Can you work these out from the model? Positions are in its coordinate system, mm. Give positions to 0.01 mm unless a question says otherwise; leave off trailing zeros. Order: outer loops, then holes, each group sorted by start corner. A loop starts at its lowest first (then second) coordinate and runs counter-clockwise, first axis right, second up. Notation, with made-up numbers: (51, 2.25) -> (66, 2.25) arc R14 cw to (66, 15.25) -> close; hole circle Ø11 at (33.5, -26). An arc over 180 degrees is marked (long way). Answer as a JSON object with one key per item and string values.
```python
from build123d import *

# Parameters (mm, degrees)
SKETCH_1_R          = 1.5
EXTRUDE_1_DEPTH     = 2
FILLET_2_R          = 5
FILLET_3_R          = 5
SKETCH_7_R          = 6
CUT_EXTRUDE_4_DEPTH = 10
FILLET_5_R          = 5
SKETCH_8_W          = 10
SKETCH_8_H          = 2
EXTRUDE_3_DEPTH     = 12
SKETCH_9_R          = 1.5
CUT_EXTRUDE_5_DEPTH = 12
FILLET_6_R          = 2
SKETCH_10_W         = 10
SKETCH_10_H         = 2
EXTRUDE_4_DEPTH     = 14
FILLET_7_R          = 5
FILLET_8_R          = 5


with BuildPart() as part:
    # 草图1 → 凸台-拉伸1 (new body)
    with BuildSketch(Plane(origin=(0, 0, 0), x_dir=(1, 0, 0), z_dir=(0, 1, 0))):
        with BuildLine():
            Line((17.196152423, -13), (52, -13))
            Line((52, -13), (52, -5.5))
            Line((52, -5.5), (-15, -5.5))
            Line((-15, -5.5), (-15, 5))
            Line((-15, 5), (-25, 5))
            Line((-25, 5), (-25, -13))
            Line((-25, -13), (6.803847577, -13))
            ThreePointArc((6.803847577, -13), (12, -16), (17.196152423, -13))
        make_face()
        with Locations(Location((-20, 0, 0), (0, 0, 270))):
            Circle(SKETCH_1_R, mode=Mode.SUBTRACT)
    extrude(amount=EXTRUDE_1_DEPTH)

    # 圆角2
    fillet_2_edges = [part.edges().sort_by_distance(p)[0] for p in [
        (-25, 1, -5),
    ]]
    fillet(fillet_2_edges, radius=FILLET_2_R)

    # 圆角3
    fillet_3_edges = [part.edges().sort_by_distance(p)[0] for p in [
        (-25, 1, 13),
    ]]
    fillet(fillet_3_edges, radius=FILLET_3_R)

    # 草图7 → 切除-拉伸4 (cut)
    with BuildSketch(Plane(origin=(0, 2, 0), x_dir=(1, 0, 0), z_dir=(0, 1, 0))):
        with Locations((12, -2.5)):
            Circle(SKETCH_7_R)
    extrude(amount=-CUT_EXTRUDE_4_DEPTH, mode=Mode.SUBTRACT)

    # 圆角5
    fillet_5_edges = [part.edges().sort_by_distance(p)[0] for p in [
        (17.196152423, 1, 13),
        (6.803847577, 1, 13),
        (6.803847577, 1, 5.5),
        (17.196152423, 1, 5.5),
    ]]
    fillet(fillet_5_edges, radius=FILLET_5_R)

    # 草图8 → 凸台-拉伸3 (add)
    with BuildSketch(Plane.XY.offset(13)):
        with Locations((47, 1)):
            Rectangle(SKETCH_8_W, SKETCH_8_H)
    extrude(amount=EXTRUDE_3_DEPTH)

    # 草图9 → 切除-拉伸5 (cut)
    with BuildSketch(Plane(origin=(0, 2, 0), x_dir=(1, 0, 0), z_dir=(0, 1, 0))):
        with Locations(Location((47, -19, 0), (0, 0, 270))):
            Circle(SKETCH_9_R)
    extrude(amount=-CUT_EXTRUDE_5_DEPTH, mode=Mode.SUBTRACT)

    # 圆角6
    fillet_6_edges = [part.edges().sort_by_distance(p)[0] for p in [
        (52, 1, 5.5),
        (52, 1, 25),
        (42, 1, 25),
    ]]
    fillet(fillet_6_edges, radius=FILLET_6_R)

    # 草图10 → 凸台-拉伸4 (add)
    with BuildSketch(Plane(origin=(-15, 0, 0), x_dir=(0, 0, -1), z_dir=(1, 0, 0))):
        with Locations((0, 1)):
            Rectangle(SKETCH_10_W, SKETCH_10_H)
    extrude(amount=EXTRUDE_4_DEPTH)

    # 圆角7
    fillet_7_edges = [part.edges().sort_by_distance(p)[0] for p in [
        (-1, 1, 5),
    ]]
    fillet(fillet_7_edges, radius=FILLET_7_R)

    # 圆角8
    fillet_8_edges = [part.edges().sort_by_distance(p)[0] for p in [
        (-1, 1, -5),
    ]]
    fillet(fillet_8_edges, radius=FILLET_8_R - 0.0001)  # a hair under: the kernel refuses the full size


solid = part.part
```
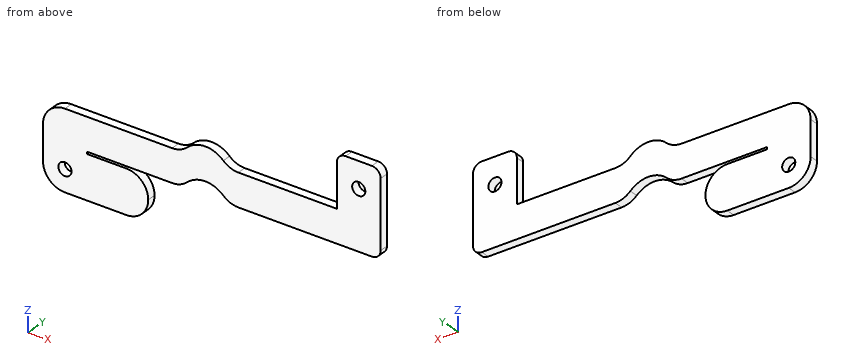
1. If we section it at A-A on x = -10: Please give me the cut outline in (y, z), then the cut area to 3 significant figures.
Worked answers:
{"outline": "(0, -5) -> (2, -5) -> (2, 5) -> (0, 5) -> close; (0, 5.5) -> (2, 5.5) -> (2, 13) -> (0, 13) -> close", "area": "35.0 mm²"}
2. If we section it at D-D on x = 34: Please give me the cut outline in (y, z).
Worked answers:
{"outline": "(0, 5.5) -> (2, 5.5) -> (2, 13) -> (0, 13) -> close"}
3. If we section it at C-C on y = 1.7: Count the separate pieces of the cut face and the enclosed holes in it, then the cut area to 3 significant figures.
Worked answers:
{"separate pieces": "1", "enclosed holes": "2", "area": "904 mm²"}
4. Please list where these lines run through material, in increasing order: L1, parallel to X at y = 1.3, z = 19; L2, parallel to X at y = 1.6, z = 20.75; L3, parallel to X at y = 1.4, z = 18.5.
Worked answers:
{"L1": "42 to 45.5, 48.5 to 52", "L2": "42 to 52", "L3": "42 to 45.59, 48.41 to 52"}
5. Will these pins go through, and if not, where does the flat tip stop? pin 1 Ø1 at (y, z) = (1, 20.5) entering from -X; pin 2 Ø0.6 at (x, y) = (-5.5, 1) entering from +Z; pin 3 Ø2.5 at (x, z) = (47, 19) entering from -Y.
Worked answers:
{"pin 1": "x = 42", "pin 2": "z = 13", "pin 3": "through"}
6. If we section it at B-B on z = 19: Please give me the cut outline in (x, y).
Worked answers:
{"outline": "(42, 0) -> (45.5, 0) -> (45.5, 2) -> (42, 2) -> close; (48.5, 0) -> (52, 0) -> (52, 2) -> (48.5, 2) -> close"}
